The listing builds one solid part. Answer for the finished solid, in the listing's coordinates (mm). A direction names the side the tool comes from. Give positions to 0.01 mm unless a question says otherwise; leave off trailing zeros. Order: outer loops, then holes, each group sorted by start corner. A loop starts at its lowest first (then second) coordinate and runs counter-clockwise, first axis right, second up.
```python
from build123d import *

# Parameters (mm, degrees)
SKETCH_1_R          = 10.5
EXTRUDE_1_DEPTH     = 5.2
SKETCH_2_R          = 1.9
CUT_EXTRUDE_1_DEPTH = 16.733403955
EXTRUDE_START       = 1
SKETCH_3_R          = 4
SKETCH_3_R_2        = 1.9
EXTRUDE_2_DEPTH     = 1
SKETCH_4_R          = 0.771394001
CUT_EXTRUDE_3_DEPTH = 16.733403955


with BuildPart() as part:
    # Эскиз1 → Бобышка-Вытянуть1 (new body)
    with BuildSketch(Plane(origin=(0, 0, 0), x_dir=(1, 0, 0), z_dir=(0, 1, 0))):
        with Locations(Location((0, 0, 0), (0, 0, 270))):
            Circle(SKETCH_1_R)
    extrude(amount=EXTRUDE_1_DEPTH)

    # Эскиз2 → Вырез-Вытянуть1 (cut, through all)
    with BuildSketch(Plane(origin=(0, 5.2, 0), x_dir=(1, 0, 0), z_dir=(0, 1, 0))):
        with Locations(Location((0, 0, 0), (0, 0, 270))):
            Circle(SKETCH_2_R)
    extrude(amount=-CUT_EXTRUDE_1_DEPTH, mode=Mode.SUBTRACT)

    # Эскиз3 → Бобышка-Вытянуть2 (add)
    with BuildSketch(Plane(origin=(0, 5.2, 0), x_dir=(1, 0, 0), z_dir=(0, 1, 0)).offset(EXTRUDE_START)):
        with Locations(Location((0, 0, 0), (0, 0, 270))):
            Circle(SKETCH_3_R)
        with Locations(Location((0, 0, 0), (0, 0, 270))):
            Circle(SKETCH_3_R_2, mode=Mode.SUBTRACT)
    extrude(amount=-EXTRUDE_2_DEPTH)

    # Эскиз4 → Вырез-Вытянуть3 (cut, through all)
    with BuildSketch(Plane(origin=(0, 5.2, 0), x_dir=(1, 0, 0), z_dir=(0, 1, 0))):
        with Locations((0, 10.5)):
            Circle(SKETCH_4_R)
        with Locations((2.183072754, 10.270549808)):
            Circle(SKETCH_4_R)
        with Locations((4.270734752, 9.592227305)):
            Circle(SKETCH_4_R)
        with Locations((6.171745149, 8.494678441)):
            Circle(SKETCH_4_R)
        with Locations((7.803020668, 7.025871367)):
            Circle(SKETCH_4_R)
        with Locations((9.09326674, 5.25)):
            Circle(SKETCH_4_R)
        with Locations((9.986093421, 3.244678441)):
            Circle(SKETCH_4_R)
        with Locations((10.442479901, 1.097548864)):
            Circle(SKETCH_4_R)
        with Locations((10.442479901, -1.097548864)):
            Circle(SKETCH_4_R)
        with Locations((9.986093421, -3.244678441)):
            Circle(SKETCH_4_R)
        with Locations((9.09326674, -5.25)):
            Circle(SKETCH_4_R)
        with Locations((7.803020668, -7.025871367)):
            Circle(SKETCH_4_R)
        with Locations((6.171745149, -8.494678441)):
            Circle(SKETCH_4_R)
        with Locations((4.270734752, -9.592227305)):
            Circle(SKETCH_4_R)
        with Locations((2.183072754, -10.270549808)):
            Circle(SKETCH_4_R)
        with Locations((0, -10.5)):
            Circle(SKETCH_4_R)
        with Locations((-2.183072754, -10.270549808)):
            Circle(SKETCH_4_R)
        with Locations((-4.270734752, -9.592227305)):
            Circle(SKETCH_4_R)
        with Locations((-6.171745149, -8.494678441)):
            Circle(SKETCH_4_R)
        with Locations((-7.803020668, -7.025871367)):
            Circle(SKETCH_4_R)
        with Locations((-9.09326674, -5.25)):
            Circle(SKETCH_4_R)
        with Locations((-9.986093421, -3.244678441)):
            Circle(SKETCH_4_R)
        with Locations((-10.442479901, -1.097548864)):
            Circle(SKETCH_4_R)
        with Locations((-10.442479901, 1.097548864)):
            Circle(SKETCH_4_R)
        with Locations((-9.986093421, 3.244678441)):
            Circle(SKETCH_4_R)
        with Locations((-9.09326674, 5.25)):
            Circle(SKETCH_4_R)
        with Locations((-7.803020668, 7.025871367)):
            Circle(SKETCH_4_R)
        with Locations((-6.171745149, 8.494678441)):
            Circle(SKETCH_4_R)
        with Locations((-4.270734752, 9.592227305)):
            Circle(SKETCH_4_R)
        with Locations((-2.183072754, 10.270549808)):
            Circle(SKETCH_4_R)
    extrude(amount=-CUT_EXTRUDE_3_DEPTH, mode=Mode.SUBTRACT)


solid = part.part
```
1) A tool of negligible diameter and unlimited length cuts with its end or side. For faces 1 (the cylindrical face through (0.02, 2.64, 9.73)), 2 (the cylindrical face through (-3.905, 5.707, -0.867)), from which of +Z, -Z, +X, -X, +Y, -Y can it reach the whole face along a straight path? Write none if from no direction.
Geometry says:
face 1: +Z, +Y, -Y
face 2: +Y
2) Find section B-B (x = 0). Write down the section's boundary in (y, z).
Geometry says:
outline: (0, -9.73) - (5.2, -9.73) - (5.2, -4) - (6.2, -4) - (6.2, -1.9) - (0, -1.9) - close; (0, 1.9) - (6.2, 1.9) - (6.2, 4) - (5.2, 4) - (5.2, 9.73) - (0, 9.73) - close
3) Find section C-C (y = 5.75). Write down the section's boundary in (x, z), then the cut area to 3 significant figures.
Geometry says:
outline: circle Ø8 at (0, 0); hole circle Ø3.8 at (0, 0)
area: 38.9 mm2
4) Given P1, Ø10, axis at x = 7.5, z = -8, coming from the +Y side; P2, Ø1.5, axis at y = 5.5, z = 3, coming from the +X side; P3, Ø2, axis at y = 2.5, z = -4, coming from the +X side, each flat-ended and moving along its own axis, determine where each tip first touches the part or whether it passes through.
Geometry says:
P1: stops at y = 5.2
P2: stops at x = 10.24
P3: stops at x = 9.72
5) Find section A-A (z = 0). Write down the section's boundary in (x, y).
Geometry says:
outline: (-10.5, 0) - (-1.9, 0) - (-1.9, 6.2) - (-4, 6.2) - (-4, 5.2) - (-10.5, 5.2) - close; (1.9, 0) - (10.5, 0) - (10.5, 5.2) - (4, 5.2) - (4, 6.2) - (1.9, 6.2) - close
6) Straight lines are drawn through the part: probe 1 along X at (y, z) = (4.75, 0); probe 2 along Z at (x, y) = (8.5, 3.5); probe 3 along Y at (x, z) = (-7, 5.75). For each, find the intervals that lie inside material, in ascending order.
Geometry says:
probe 1: x = -10.5 to -1.9, 1.9 to 10.5
probe 2: z = -6.16 to -5.74, -4.76 to 4.76, 5.74 to 6.16
probe 3: y = 0 to 5.2
7) Find section D-D (x = 2.5). Write down the section's boundary in (y, z), then the cut area to 3 significant figures.
Geometry says:
outline: (0, -9.57) - (5.2, -9.57) - (5.2, -3.12) - (6.2, -3.12) - (6.2, 3.12) - (5.2, 3.12) - (5.2, 9.57) - (0, 9.57) - close
area: 106 mm2
